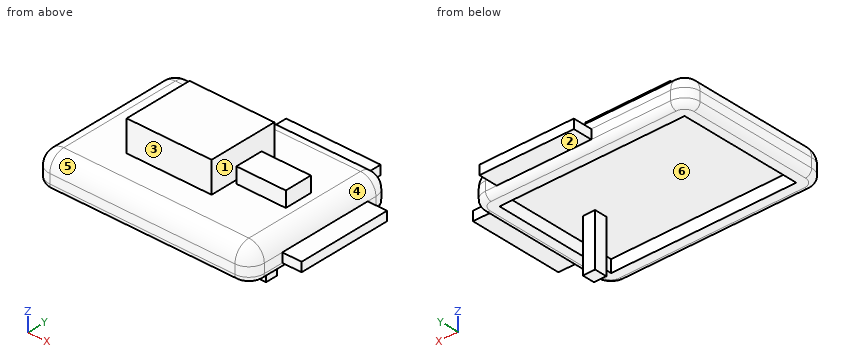
```python
from build123d import *

# Parameters (mm, degrees)
F0_W      = 177.8
F0_H      = 25.4
F1_DEPTH  = 127
F2_R      = 12.7
F3_R      = 12.7
F4_R      = 12.7
F5_W      = 152.4
F5_H      = 101.6
F6_DEPTH  = 10.16
F7_R      = 5.08
F8_W      = 10.16
F8_H      = 10.16
F9_DEPTH  = 43.18
F10_W     = 69.85
F10_H     = 57.15
F11_DEPTH = 25.4
F10_W_2   = 40.64
F10_H_2   = 22.86
F12_DEPTH = 12.7
F13_W     = 77.7875
F13_H     = 7.62
F14_DEPTH = 15.875
F15_W     = 77.7875
F15_H     = 7.62
F16_DEPTH = 15.875


with BuildPart() as f1:
    # F0 (on Front) → F1 (new body)
    with BuildSketch(Plane.XZ):
        with Locations((6.3456185162, 8.1420660227)):
            Rectangle(F0_W, F0_H)
    extrude(amount=F1_DEPTH)

    # F2
    f2_edges = [f1.edges().sort_by_distance(p)[0] for p in [
        (6.345619, -127, 20.842066),
        (-82.554381, -127, 8.142066),
        (-82.554381, -63.5, 20.842066),
    ]]
    fillet(f2_edges, radius=F2_R)

    # F3
    f3_edges = [f1.edges().sort_by_distance(p)[0] for p in [
        (95.245619, -57.15, 20.842066),
        (12.695619, -114.3, 20.842066),
        (95.245619, -127, 1.792066),
    ]]
    fillet(f3_edges, radius=F3_R)

    # F4
    f4_edges = [f1.edges().sort_by_distance(p)[0] for p in [
        (6.345619, 0, 20.842066),
        (-69.854381, -57.15, 20.842066),
        (-82.554381, 0, 1.792066),
    ]]
    fillet(f4_edges, radius=F4_R)

    # F5 (on face) → F6 (cut)
    with BuildSketch(Plane(origin=(0, 0, -4.5579339773), x_dir=(1, 0, 0), z_dir=(0, 0, -1))):
        with Locations((6.3456185162, 63.5)):
            Rectangle(F5_W, F5_H)
    extrude(amount=-F6_DEPTH, mode=Mode.SUBTRACT)

    # F7
    f7_edges = [f1.edges().sort_by_distance(p)[0] for p in [
        (6.345619, -127, -4.557934),
        (95.245619, -63.5, -4.557934),
        (91.525875, -123.280256, -4.557934),
    ]]
    fillet(f7_edges, radius=F7_R)

    # F8 (on face) → F9 (join)
    with BuildSketch(Plane(origin=(0, 0, 5.6020660227), x_dir=(1, 0, 0), z_dir=(0, 0, -1))):
        with Locations((57.6618951797, 71.7390547824)):
            Rectangle(F8_W, F8_H)
    extrude(amount=F9_DEPTH)

    # F10 (on face) → F11 (join)
    with BuildSketch(Plane.XY.offset(20.8420660227)):
        with Locations((-2.115206793, -64.7223750857)):
            Rectangle(F10_W, F10_H)
    extrude(amount=F11_DEPTH)

    # F10 (on face) → F12 (join)
    with BuildSketch(Plane.XY.offset(20.8420660227)):
        with Locations((56.0945885849, -62.5277971399)):
            Rectangle(F10_W_2, F10_H_2)
    extrude(amount=F12_DEPTH)

    # F13 (on face) → F14 (join)
    with BuildSketch(Plane.YZ.offset(95.2456185162)):
        with Locations((-59.0517186254, 4.3320660227)):
            Rectangle(F13_W, F13_H)
    extrude(amount=F14_DEPTH)

    # F15 (on face) → F16 (join)
    with BuildSketch(Plane(origin=(0, 0, 0), x_dir=(-1, 0, 0), z_dir=(0, 1, 0))):
        with Locations((-34.4312283516, 4.3320660227)):
            Rectangle(F15_W, F15_H)
    extrude(amount=F16_DEPTH)


solid = f1.part
```
Verification items for the finished model (mm, model axes). Face numbers are marked on the shaded views. A direction names the side the tool comes from. Round coordinates to 2 decimals unless told otherwise and drop trailing zeros. Loops run counter-clockwise (first coordinate to the right, second up) from the corner with the lowest first, then second, coordinate; pieces in that order, holes last. Notation, with made-up numbers: (88, -3.5) -> (128, -3.5) arc R20 ccw to (128, 27.5) -> close; hole circle Ø1 at (76, 67.5). An arc over 180 degrees is marked (long way). Answer as a JSON object with one key per item and string values.
Q1. Section check A-A (z = 25). Record the boundary of the cut face in (x, y), then the cut area to 3 significant figures.
Data:
{"outline": "(-37.04, -93.3) -> (32.81, -93.3) -> (32.81, -36.15) -> (-37.04, -36.15) -> close; (35.77, -73.96) -> (76.41, -73.96) -> (76.41, -51.1) -> (35.77, -51.1) -> close", "area": "4,920 mm2"}
Q2. Go/stop test with flat-tipped pins: P1, Ø6.5, axis at x = 55, z = 28, coming from the -Y side; P2, Ø12, axis at x = 86, z = 18.5, coming from the -Y side; P3, Ø5, axis at x = 38.5, y = 6.5, coming from the +Z side; P4, Ø8, axis at x = 31.5, z = -1, coming from the -Y side. Record where each tip stops, or that it passes through.
Data:
{"P1": "stops at y = -73.96", "P2": "stops at y = -126.01", "P3": "stops at z = 8.14", "P4": "stops at y = -127"}
Q3. Scan lines: line 1 (Y direction, x = 1, z = 28); line 2 (Z direction, x = -0.5, y = -51); line 3 (Z direction, x = -14, y = -108). Record each from-to range of solid material in increasing order. Write a range as from..to.
Data:
{"line 1": "y = -93.3..-36.15", "line 2": "z = 5.6..46.24", "line 3": "z = 5.6..20.84"}
Q4. Section check B-B (x = -2). Record the boundary of the cut face in (y, z) (3 decimals), then the cut area to 3 significant figures.
Data:
{"outline": "(-127, 0.522) arc R5.08 ccw to (-121.92, -4.558) -> (-114.3, -4.558) -> (-114.3, 5.602) -> (-12.7, 5.602) -> (-12.7, -4.558) -> (-5.08, -4.558) arc R5.08 ccw to (0, 0.522) -> (15.875, 0.522) -> (15.875, 8.142) -> (0, 8.142) arc R12.7 ccw to (-12.7, 20.842) -> (-36.147, 20.842) -> (-36.147, 46.242) -> (-93.297, 46.242) -> (-93.297, 20.842) -> (-114.3, 20.842) arc R12.7 ccw to (-127, 8.142) -> close", "area": "3,690 mm2"}
Q5. Draft check along Y on the marked faces 4, 5 and 6. Enter one of: pulls with the +Y half, pulls with the -Y half, needs draft (parallel to the pull), parting line crosses it, or undercut.
Data:
{"face 4": "needs draft", "face 5": "pulls with the -Y half", "face 6": "undercut"}
Q6. Section check D-D (y = -60). Record the boundary of the cut face in (x, z).
Data:
{"outline": "(-82.55, 0.52) arc R5.08 ccw to (-77.47, -4.56) -> (-69.85, -4.56) -> (-69.85, 5.6) -> (82.55, 5.6) -> (82.55, -4.56) -> (90.17, -4.56) arc R5.08 ccw to (95.25, 0.52) -> (111.12, 0.52) -> (111.12, 8.14) -> (95.25, 8.14) arc R12.7 ccw to (82.55, 20.84) -> (76.41, 20.84) -> (76.41, 33.54) -> (35.77, 33.54) -> (35.77, 20.84) -> (32.81, 20.84) -> (32.81, 46.24) -> (-37.04, 46.24) -> (-37.04, 20.84) -> (-69.85, 20.84) arc R12.7 ccw to (-82.55, 8.14) -> close"}
Q7. Section check C-C (y = -107). Record the boundary of the cut face in (x, z), then the cut area to 3 significant figures.
Data:
{"outline": "(-82.55, 0.52) arc R5.08 ccw to (-77.47, -4.56) -> (-69.85, -4.56) -> (-69.85, 5.6) -> (82.55, 5.6) -> (82.55, -4.56) -> (90.17, -4.56) arc R5.08 ccw to (95.25, 0.52) -> (95.25, 8.14) arc R12.7 ccw to (82.55, 20.84) -> (-69.85, 20.84) arc R12.7 ccw to (-82.55, 8.14) -> close", "area": "2,890 mm2"}
Q8. Access from +Z, -Z, +X, -X, +Y, -Y to the whole of each face (thin tool, end or side, straight path). Record for the marked faces 1, 2 and 3.
Data:
{"face 1": "+Z, +Y, -Y", "face 2": "-Z, +X, -X, +Y", "face 3": "+Z, +X, -X, -Y"}
